Autodesk Inventor part; units mm, degrees
ref_plane "YZ Plane" through (0, 0, 0) normal (1, 0, 0) x (0, 1, 0)
ref_plane "XZ Plane" through (0, 0, 0) normal (0, 1, 0) x (-1, 0, 0)
ref_plane "XY Plane" through (0, 0, 0) normal (0, 0, 1) x (1, 0, 0)
sketch "FSM2JH, Pushbutton_60" plane through (0, 0, 0) normal (0, 0, 1) x (1, 0, 0)
  line L0 (1.6251, 0.2499) -> (4.3749, 0.2499)
  arc A0 (4.3749, 0.2499) -> (5.125, 1) centre (4.3749, 1) ccw
  line L1 (5.125, 1) -> (5.125, 3.5001)
  arc A1 (5.125, 3.5001) -> (4.3749, 4.2499) centre (4.375, 3.5) ccw
  line L2 (4.3749, 4.2499) -> (1.6251, 4.2499)
  arc A2 (1.6251, 4.2499) -> (0.875, 3.5001) centre (1.625, 3.5) ccw
  line L3 (0.875, 3.5001) -> (0.875, 1)
  arc A3 (0.875, 1) -> (1.6251, 0.2499) centre (1.6251, 1) ccw
extrude "Extrusion1" add sketch "FSM2JH, Pushbutton_60" along normal blind 6.35
properties part number "Pushbutton"
The model under review builds one solid part; all positions refer to its coordinate system, in mm. Coordinates: 2 decimals unless noted, no trailing zeros. Write each loop counter-clockwise with the first axis right and the second up, starting at its lowest first coordinate (ties: lowest second). Pieces come first, ordered by that corner, then holes. Notation, with made-up numbers: (3.25, 27.25) - (14.25, 27.25) arc R35 cw to (14.25, 64.25) - close; hole circle Ø1 at (48, -9.75). An arc over 180 degrees is marked (long way). Answer in a Markdown table with one row per item. Add a question column.
Q1. Consider section A-A on z = 0.75. Give the boundary of the cut face in (x, y) (3 decimals), then the cut area to 3 significant figures.
Q2. Consider section C-C on y = 3.8. Give the boundary of the cut face in (x, z).
Q3. Consider section B-B on x = 1.1. Give the boundary of the cut face in (y, z), then the cut area to 3 significant figures.
Q4. Clearance check with a flat-ended pin moving along its axis: pin 1 (2 mm diameter, centred on x = 2.5, y = 1, fed in from -Z). State where the tip first meets the part, or that it passes through.
Q5. To check wall thickness, follow line 1 along Y through (x, z) = (1.25, 1.25); line 2 along Y through (x, z) = (4.45, 2.25); line 3 along X through (y, z) = (0.7, 2). State the ranges of each line that lie inside material, in increasing order. Write a range as from..to.
Answers below:
| question | item | result |
|---|---|---|
| 1 | outline | (0.875, 1) arc R0.75 ccw to (1.625, 0.25) - (4.375, 0.25) arc R0.75 ccw to (5.125, 1) - (5.125, 3.5) arc R0.75 ccw to (4.375, 4.25) - (1.625, 4.25) arc R0.75 ccw to (0.875, 3.5) - close |
| 1 | area | 16.5 mm² |
| 2 | outline | (0.94, 0) - (5.06, 0) - (5.06, 6.35) - (0.94, 6.35) - close |
| 3 | outline | (0.46, 0) - (4.04, 0) - (4.04, 6.35) - (0.46, 6.35) - close |
| 3 | area | 22.7 mm² |
| 4 | pin 1 | z = 0 |
| 5 | line 1 | 0.35..4.15 |
| 5 | line 2 | 0.25..4.25 |
| 5 | line 3 | 0.94..5.06 |
